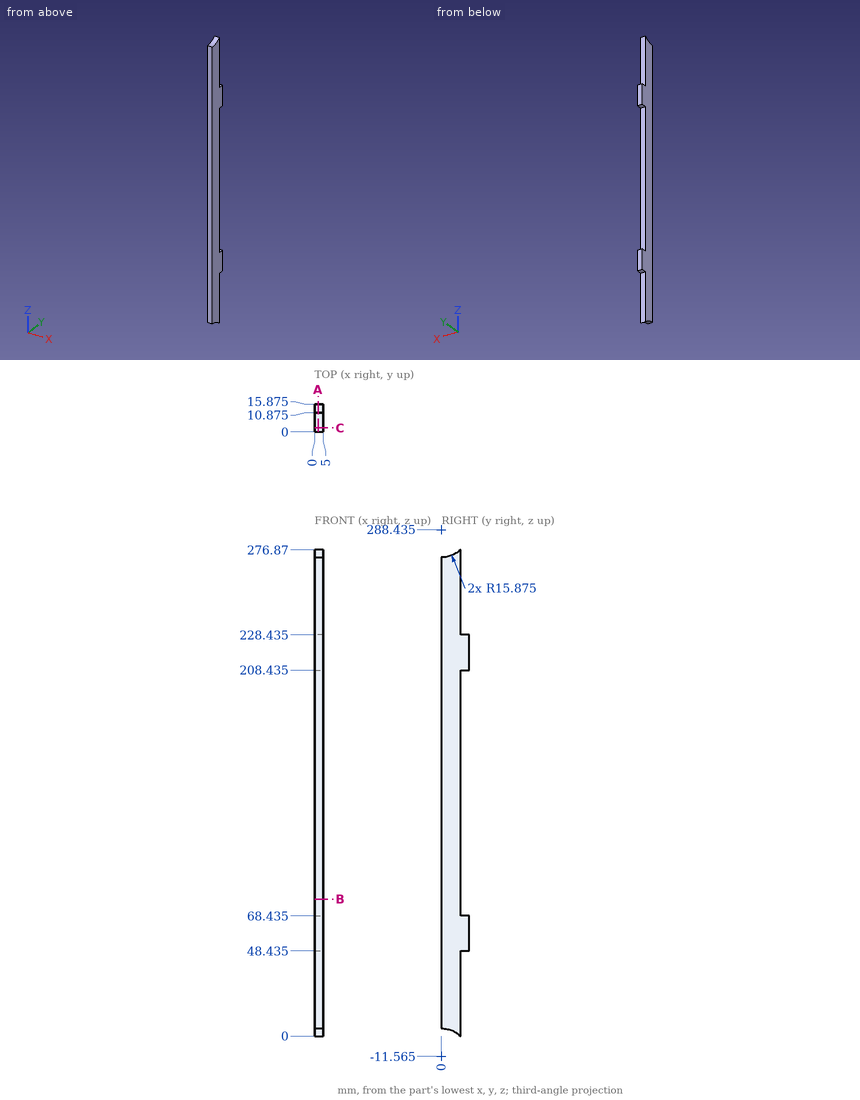
Answer from the drawing. Dimensions are ordinates in mm from the lowest x, y and z of the part. Round coordinates to 2 decimals unless told otherwise and drop trailing zeros. Write each loop counter-clockwise with the first axis right and the second up, starting at its lowest first coordinate (ties: lowest second). Pieces come first, ordered by that corner, then holes.
1. The part is cut by section C-C, the plane y = 2.25. Determine the outline of the cut face in (x, z).
2. Given pin 1 Ø2.5 at (x, y) = (2, 14.5) entering from -Z (3 decimals); pin 2 Ø2.5 at (x, y) = (1.5, 14) entering from +Z (3 decimals); pin 3 Ø1 at (x, z) = (2, 93) entering from +Y (3 decimals); pin 4 Ø5 at (y, z) = (14, 146) entering from -X, each flat-ended and moving along its own axis, determine where each tip first touches the part or whether it passes through.
3. The part is cut by section B-B, the plane z = 78. Determine the outline of the cut face in (x, y) (3 decimals).
4. Straight lines are drawn through the part: L1, parallel to Z at x = 3.15, y = 14.75 (3 decimals); L2, parallel to Y at x = 3.35, z = 81 (3 decimals); L3, parallel to Z at x = 3.65, y = 1. For each, find the intervals that lie inside material, in ascending order.
5. The part is cut by section A-A, the plane x = 1.9. Determine the outline of the cut face in (y, z) (3 decimals).
Values:
1. outline: (0, 4.15) - (5, 4.15) - (5, 272.72) - (0, 272.72) - close
2. pin 1: stops at z = 48.435
2. pin 2: stops at z = 228.435
2. pin 3: stops at y = 10.875
2. pin 4: passes through
3. outline: (0, 0) - (5, 0) - (5, 10.875) - (0, 10.875) - close
4. L1: z = 48.435 to 68.435, 208.435 to 228.435
4. L2: y = 0 to 10.875
4. L3: z = 4.28 to 272.59
5. outline: (0, 4.31) arc R15.875 cw to (10.875, 0) - (10.875, 48.435) - (15.875, 48.435) - (15.875, 68.435) - (10.875, 68.435) - (10.875, 208.435) - (15.875, 208.435) - (15.875, 228.435) - (10.875, 228.435) - (10.875, 276.87) arc R15.875 cw to (0, 272.56) - close
